from build123d import *

# Parameters (mm, degrees)
F1_DEPTH  = 9.525
F2_R      = 5.55625
F2_R_2    = 6.35
F3_DEPTH  = 2.38125
F4_R      = 3.175
F4_R_2    = 1.8288
F4_R_3    = 1.5875
F5_DEPTH  = 5.55625
F6_R      = 2.38125
F7_DEPTH  = 1.5875
F8_SIZE   = 3.17499
F9_R      = 3.175
F10_DEPTH = 3.175


# Not quite as in the source:
# - a fillet or chamfer is up to 0.001 mm smaller than in the source, because OpenCascade refuses the exact size


with BuildPart() as f1:
    # F0 (on Top) → F1 (new body)
    with BuildSketch(Plane.XY):
        Polygon((0, 0), (0, 55.7060608), (-2.38125, 55.7060608), (-2.38125, 49.3560608), (-5.55625, 49.3560608), (-5.55625, 39.8310608), (-2.38125, 39.8310608), (-2.38125, 15.875), (-5.55625, 15.875), (-5.55625, 6.35), (-2.38125, 6.35), (-2.38125, 0), align=None)
    extrude(amount=F1_DEPTH)

    # F2 (on face) → F3 (join, through all)
    with BuildSketch(Plane(origin=(-2.38125, 0, 0), x_dir=(0, -1, 0), z_dir=(-1, 0, 0))):
        with Locations((-55.7060608, 4.7625)):
            Circle(F2_R)
        with Locations((0, 4.7625)):
            Circle(F2_R_2)
    extrude(amount=-F3_DEPTH)

    # F4 (on face) → F5 (cut, through all)
    with BuildSketch(Plane.YZ):
        with Locations((0, 4.7625)):
            Circle(F4_R)
        with Locations((11.1125, 4.7625)):
            Circle(F4_R_2)
        with Locations((44.5935608, 4.7625)):
            Circle(F4_R_2)
        with Locations((55.7060608001, 4.7625)):
            Circle(F4_R_3)
    extrude(amount=-F5_DEPTH, mode=Mode.SUBTRACT)

    # F6 (on face) → F7 (cut)
    with BuildSketch(Plane(origin=(-2.38125, 0, 0), x_dir=(0, -1, 0), z_dir=(-1, 0, 0))):
        with Locations((-55.7060608, 4.7625)):
            Circle(F6_R)
    extrude(amount=-F7_DEPTH, mode=Mode.SUBTRACT)

    # F8 (size 3.175 in the source; OpenCascade refuses exactly that, so slightly less here)
    f8_edges = [f1.edges().sort_by_distance(p)[0] for p in [
        (-2.38125, 39.831061, 4.7625),
        (-2.38125, 15.875, 4.7625),
    ]]
    chamfer(f8_edges, length=F8_SIZE)

    # F9 (on face) → F10 (cut)
    with BuildSketch(Plane.YZ):
        with Locations((11.1125, 4.7625)):
            Circle(F9_R)
        with Locations((44.5935608, 4.7625)):
            Circle(F9_R)
    extrude(amount=-F10_DEPTH, mode=Mode.SUBTRACT)


solid = f1.part
Part model, mm, in its own coordinate system. A direction names the side the tool comes from. Give positions to 0.01 mm unless a question says otherwise; leave off trailing zeros. Loops run counter-clockwise (first coordinate to the right, second up) from the corner with the lowest first, then second, coordinate; pieces in that order, holes last. Notation, with made-up numbers: (-40, 56) -> (9, 56) arc R17 cw to (9, 65) -> close; hole circle Ø7 at (42.5, 32). An arc over 180 degrees is marked (long way). Write each question's results on one line, items separated by ' | '. Start each with the question number.
Q1. Band-saw the part on A-A on y = 0. List the corners of the cut face in (x, z), plus the area to 3 significant figures.
Q2. Pull direction Y, two halves, no side cores. Call faces 4 (the face through (-4, 6.35, 5)), 5 (the face through (-5.556, 42.5, 4.7)), 6 (the face through (-1.599, 57.596, 3.314)): +Y half, -Y half, draft (parallel to the pull), parting line (faces both ways), or undercut.
Q3. Wall check: L1, parallel to Y at x = -2.6, z = 4; L2, parallel to Y at x = -1.8, z = 2 (1 decimal); L3, parallel to Z at x = -1.95, y = 42 (3 decimals). Give the ranges that are in metal, low to high.
Q4. Band-saw the part on B-B on x = -1.65. Count the separate pieces of the cut face and the enclosed holes in it, plus the area to 3 significant figures.
Q5. Pin check, flat tips, straight feed: P1, Ø4, axis at y = 55.71, z = 4.76, coming from the -X side; P2, Ø6, axis at y = 6, z = 4.5, coming from the -X side; P3, Ø4, axis at y = 11.11, z = 4.76, coming from the +X side (3 decimals); P4, Ø1.6, axis at x = -4, z = 5.5, coming from the -Y side. Stop position of each tip, or through.
Q6. Band-saw the part on C-C on y = 30. List the corners of the cut face in (x, z) (3 decimals), plus the area to 3 significant figures.
Q7. Band-saw the part on D-D on y = 17.5. List the corners of the cut face in (x, z) (3 decimals), plus the area to 3 significant figures.
Q8. Which spindle directions (+Z, -Z, +X, -X, +Y, -Y) get a long thin tool onto all of the face, cutting with end or side? Do faces 1 (the face through (-2.381, 3, 3)), 2 (the face through (-2, 29, 9.525)), 3 (the face through (-2.381, 28, 5)). Say none if no direction does.
Results are:
1) outline: (-2.38, -1.59) -> (0, -1.59) -> (0, 1.59) -> (-2.38, 1.59) -> close; (-2.38, 7.94) -> (0, 7.94) -> (0, 11.11) -> (-2.38, 11.11) -> close | area: 15.1 mm²
2) face 4: -Y half | face 5: draft | face 6: undercut
3) L1: y = 6.35 to 8.03, 14.19 to 18.83, 36.87 to 41.51, 47.68 to 49.36 | L2: y = -5.7 to -1.6, 1.6 to 9.5, 12.7 to 43, 46.2 to 60.5 | L3: z = 0 to 2.931, 6.594 to 9.525
4) separate pieces: 1 | enclosed holes: 4 | area: 542 mm²
5) P1: stops at x = -0.79 | P2: stops at x = -5.56 | P3: stops at x = -3.175 | P4: stops at y = 6.35
6) outline: (-2.381, 0) -> (0, 0) -> (0, 9.525) -> (-2.381, 9.525) -> close | area: 22.7 mm²
7) outline: (-3.931, 0) -> (0, 0) -> (0, 9.525) -> (-3.931, 9.525) -> close | area: 37.4 mm²
8) face 1: +Z, -Z, -X, -Y | face 2: +Z, +X, -X | face 3: +Z, -Z, -X
